```python
from build123d import *

# Parameters (mm, degrees)
F0_R     = 6.528915
F1_DEPTH = 5.08


with BuildPart() as f1:
    # F0 (on Front) → F1 (new body)
    with BuildSketch(Plane.XZ):
        with BuildLine():
            ThreePointArc((0, 5.08), (1.487898, 1.487898), (5.08, 0))
            Line((5.08, 0), (198.12, 0))
            ThreePointArc((198.12, 0), (201.712102, 1.487898), (203.2, 5.08))
            Line((203.2, 5.08), (203.2, 15.24))
            ThreePointArc((203.2, 15.24), (201.712102, 18.832102), (198.12, 20.32))
            Line((198.12, 20.32), (5.08, 20.32))
            ThreePointArc((5.08, 20.32), (1.487898, 18.832102), (0, 15.24))
            Line((0, 15.24), (0, 5.08))
        make_face()
        with Locations((12.7, 10.16)):
            Circle(F0_R, mode=Mode.SUBTRACT)
        with Locations((38.1, 10.16)):
            Circle(F0_R, mode=Mode.SUBTRACT)
        with Locations((63.5, 10.16)):
            Circle(F0_R, mode=Mode.SUBTRACT)
        with Locations((88.9, 10.16)):
            Circle(F0_R, mode=Mode.SUBTRACT)
        with Locations((114.3, 10.16)):
            Circle(F0_R, mode=Mode.SUBTRACT)
        with Locations((139.7, 10.16)):
            Circle(F0_R, mode=Mode.SUBTRACT)
        with Locations((165.1, 10.16)):
            Circle(F0_R, mode=Mode.SUBTRACT)
        with Locations((190.5, 10.16)):
            Circle(F0_R, mode=Mode.SUBTRACT)
    extrude(amount=F1_DEPTH)


solid = f1.part
```
Can you work these out from the model? Positions are in its coordinate system, mm. Round coordinates to 2 decimals unless told otherwise and drop trailing zeros. Loops run counter-clockwise (first coordinate to the right, second up) from the corner with the lowest first, then second, coordinate; pieces in that order, holes last.
Item 1: Will these pins go through, and if not, where does the flat tip stop? pin 1 Ø10.5 at (x, z) = (165.1, 10.16) entering from -Y; pin 2 Ø1 at (y, z) = (-4.5, 17.5) entering from +X.
Item 2: Suppose I cut it at B-B, the plane y = -1.5. State how many separate pieces and enclosed holes the cut face has, then the cut area to 3 significant figures.
Item 3: Suppose I cut it at A-A, the plane x = 88.9. Write out the boundary of the cut face in (y, z).
Item 4: Suppose I cut it at D-D, the plane x = 137.5. Write out the boundary of the cut face in (y, z).
Item 5: Please list where these lines run through material, in increasing order: L1, parallel to Z at x = 63.5, y = -3.1; L2, parallel to Z at x = 93, y = -2.1; L3, parallel to X at y = -1.5, z = 17.25.
Item 6: If we mould it in two halves opening along X, with no side actions, what happens to faces 1 (the flat face through (100, 0, 10)), 2 (the cylindrical face through (18.73, -2.5, 7.66)), 3 (the cylindrical face through (1.528, -2.504, 18.871))? For each: +X half, -X half, draft (parallel to the pull), parting line (faces both ways), or undercut.
Reported:
1. pin 1: passes through
1. pin 2: stops at x = 202.89
2. separate pieces: 1
2. enclosed holes: 8
2. area: 3,040 mm2
3. outline: (-5.08, 0) - (0, 0) - (0, 3.63) - (-5.08, 3.63) - close; (-5.08, 16.69) - (0, 16.69) - (0, 20.32) - (-5.08, 20.32) - close
4. outline: (-5.08, 0) - (0, 0) - (0, 4.01) - (-5.08, 4.01) - close; (-5.08, 16.31) - (0, 16.31) - (0, 20.32) - (-5.08, 20.32) - close
5. L1: z = 0 to 3.63, 16.69 to 20.32
5. L2: z = 0 to 5.08, 15.24 to 20.32
5. L3: x = 0.41 to 202.79
6. face 1: draft
6. face 2: undercut
6. face 3: -X half
